Work out the finished part from the listing and answer in its coordinate system (mm). Round coordinates to 2 decimals unless told otherwise and drop trailing zeros. One line per item, written item: value.
```python
from build123d import *

# Parameters (mm, degrees)
SKETCH1_W               = 12.7
SKETCH1_H               = 58.674
BOSS_EXTRUDE1_DEPTH     = 319.024
F_1_4_20_TAPPED_HOLE1_D = 5.1054


with BuildPart() as part:
    # Sketch1 → Boss-Extrude1 (new body)
    with BuildSketch(Plane(origin=(0, 0, 0), x_dir=(1, 0, 0), z_dir=(0, 1, 0))):
        with Locations((6.35, 29.337)):
            Rectangle(SKETCH1_W, SKETCH1_H)
    extrude(amount=-BOSS_EXTRUDE1_DEPTH)

    # 1/4-20 Tapped Hole1 (through all)
    with Locations(Plane(origin=(0, -306.324, -19.05), x_dir=(0, 0, -1), z_dir=(-1, 0, 0))):
        with Locations((0, 0), (20.574, 0), (22.098, -287.274), (-1.524, -287.274), (22.098, -249.174), (-1.524, -249.174)):
            Hole(F_1_4_20_TAPPED_HOLE1_D / 2)


solid = part.part
```
1) The mould has two halves that part along Z. Classify faces 1 (the face through (6.439, -17.497, -19.552)), 2 (the face through (6, -157, 0)), 3 (the face through (0, -157, -29)): +Z half, -Z half, draft (parallel to the pull), parting line (faces both ways), or undercut.
Check values:
face 1: undercut
face 2: +Z half
face 3: draft
2) This flat-tipped pin is pushed along its axis until it touches: pin 1 (4.5 mm diameter, centred on y = -57.15, z = -41.148, fed in from +X). Where does it stop, or does it pass through?
Check values:
pin 1: through
3) Find the intervals of material crossed by probe 1 along Z at (x, y) = (5.75, -57.15); probe 2 along Y at (x, z) = (9.75, -41.5); probe 3 along Y at (x, z) = (3.5, -37.5), in increasing order. Write a range as from..to.
Check values:
probe 1: -58.67..-43.7, -38.6..-20.08, -14.97..0
probe 2: -319.02..-308.06, -304.59..-59.68, -54.62..-21.58, -16.52..0
probe 3: -319.02..-307.74, -304.91..0
